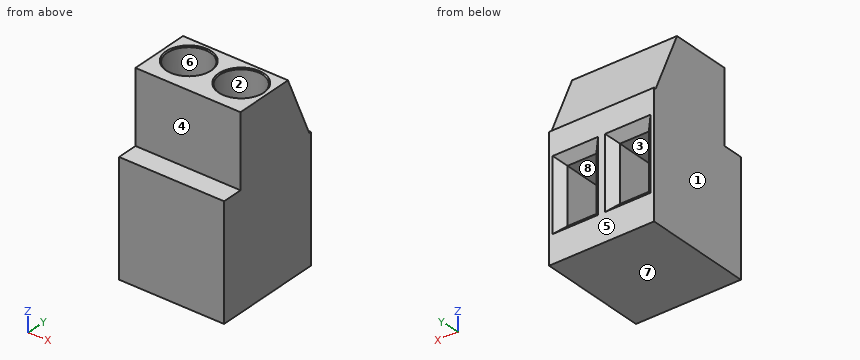
```python
from build123d import *

# Parameters (mm, degrees)
PAD_DEPTH       = 10.16
SKETCH001_R     = 2.1
POCKET_DEPTH    = 3
SKETCH002_W     = 5.4
SKETCH002_H     = 2.8
POCKET001_DEPTH = 8
CHAMFER_SIZE    = 0.8
CHAMFER001_SIZE = 0.1


with BuildPart() as part:
    # Sketch → Pad (new body)
    with BuildSketch(Plane.YZ):
        Polygon((-5.3, 0), (5.3, 0), (5.3, 12), (5.1, 12), (2.5, 18), (-3.3, 18), (-3.3, 11), (-5.3, 11), align=None)
    extrude(amount=PAD_DEPTH)

    # Sketch001 (on Face5 of Pad) → Pocket (cut)
    with BuildSketch(Plane(origin=(0, 0, 18), x_dir=(0, -1, 0), z_dir=(0, 0, 1))):
        with Locations((0, 2.54)):
            Circle(SKETCH001_R)
        with Locations((0, 7.62)):
            Circle(SKETCH001_R)
    extrude(amount=-POCKET_DEPTH, mode=Mode.SUBTRACT)

    # Sketch002 (on Face3 of Pocket) → Pocket001 (cut)
    with BuildSketch(Plane.ZX.offset(5.3)):
        with Locations((6.2, 7.62)):
            Rectangle(SKETCH002_W, SKETCH002_H)
        with Locations((6.2, 2.54)):
            Rectangle(SKETCH002_W, SKETCH002_H)
    extrude(amount=-POCKET001_DEPTH, mode=Mode.SUBTRACT)

    # Chamfer
    chamfer_edges = [part.edges().sort_by_distance(p)[0] for p in [
        (6.22, 5.3, 6.2),
        (7.62, 5.3, 8.9),
        (9.02, 5.3, 6.2),
        (7.62, 5.3, 3.5),
        (3.94, 5.3, 6.2),
        (2.54, 5.3, 8.9),
        (1.14, 5.3, 6.2),
        (2.54, 5.3, 3.5),
    ]]
    chamfer(chamfer_edges, length=CHAMFER_SIZE)

    # Chamfer001
    chamfer001_edges = [part.edges().sort_by_distance(p)[0] for p in [
        (7.62, 2.1, 18),
        (2.54, 2.1, 18),
    ]]
    chamfer(chamfer001_edges, length=CHAMFER001_SIZE)


solid = part.part
```
Geometry check sheet. Reference: the model listing, model coordinates, mm. Face numbers are marked on the shaded views. A direction names the side the tool comes from. Round coordinates to 2 decimals unless told otherwise and drop trailing zeros. Order: outer loops, then holes, each group sorted by start corner. A loop starts at its lowest first (then second) coordinate and runs counter-clockwise, first axis right, second up. Notation, with made-up numbers: (-27.5, 13) - (-10.5, 13) arc R24 cw to (-10.5, 29) - close; hole circle Ø7 at (-20, -13). An arc over 180 degrees is marked (long way). Use a Markdown table: item, result. Add a question column.
(1) Material ranges on line 1 along X through (y, z) = (-0.75, 7.5); line 2 along X through (y, z) = (0, 15.8); line 3 along Z through (x, y) = (1.25, -2.5), recorded low to high. Write a range as [from, to].
(2) Tool access check on the marked faces 1, 2, 3, 4 and 5. Record the directions out of +Z, -Z, +X, -X, +Y, -Y that give a thin tool (end or side, any length) a straight path to the whole face; none if there is none.
(3) Sectioned sample at A-A, the plane z = 4. Enter the section's corners in (x, y).
(4) Depth check by flat-ended pin: pin 1 (0.8 mm diameter, centred on x = 2, z = 6, fed in from +Y); pin 2 (0.8 mm diameter, centred on x = 2.5, y = 2, fed in from -Z); pin 3 (2 mm diameter, centred on x = 3, y = 0.5, fed in from +Z). Enter the tip coordinate at first touch or a pass-through.
(5) Sectioned sample at C-C, the plane x = 2.54. Enter the section's corners in (y, z).
(6) Sectioned sample at D-D, the plane y = -4.5. Enter the section's corners in (x, z).
(7) Sectioned sample at B-B, the plane y = 0. Enter the section's corners in (x, z).
(8) Release check for a two-part mould opening along Z. For the marked faces 6, 7 and 8 record: pulls with the +Z half, pulls with the -Z half, needs draft (parallel to the pull), parting line crosses it, or undercut.
Answers below:
| question | item | result |
|---|---|---|
| 1 | line 1 | [0, 1.14], [3.94, 6.22], [9.02, 10.16] |
| 1 | line 2 | [0, 0.44], [4.64, 5.52], [9.72, 10.16] |
| 1 | line 3 | [0, 3.5], [8.9, 18] |
| 2 | face 1 | +Z, -Z, -X, +Y, -Y |
| 2 | face 2 | +Z |
| 2 | face 3 | +Y |
| 2 | face 4 | +Z, +X, -X, -Y |
| 2 | face 5 | +Z, -Z, +X, -X, +Y |
| 3 | outline | (0, -5.3) - (10.16, -5.3) - (10.16, 5.3) - (9.82, 5.3) - (9.02, 4.5) - (9.02, -2.7) - (6.22, -2.7) - (6.22, 4.5) - (5.42, 5.3) - (4.74, 5.3) - (3.94, 4.5) - (3.94, -2.7) - (1.14, -2.7) - (1.14, 4.5) - (0.34, 5.3) - (0, 5.3) - close |
| 4 | pin 1 | y = -2.7 |
| 4 | pin 2 | z = 0 |
| 4 | pin 3 | z = 15 |
| 5 | outline | (-5.3, 0) - (5.3, 0) - (5.3, 2.7) - (4.5, 3.5) - (-2.7, 3.5) - (-2.7, 8.9) - (4.5, 8.9) - (5.3, 9.7) - (5.3, 12) - (5.1, 12) - (2.5, 18) - (2.2, 18) - (2.1, 17.9) - (2.1, 15) - (-2.1, 15) - (-2.1, 17.9) - (-2.2, 18) - (-3.3, 18) - (-3.3, 11) - (-5.3, 11) - close |
| 6 | outline | (0, 0) - (10.16, 0) - (10.16, 11) - (0, 11) - close |
| 7 | outline | (0, 0) - (10.16, 0) - (10.16, 18) - (9.82, 18) - (9.72, 17.9) - (9.72, 15) - (5.52, 15) - (5.52, 17.9) - (5.42, 18) - (4.74, 18) - (4.64, 17.9) - (4.64, 15) - (0.44, 15) - (0.44, 17.9) - (0.34, 18) - (0, 18) - close; hole (1.14, 3.5) - (3.94, 3.5) - (3.94, 8.9) - (1.14, 8.9) - close; hole (6.22, 3.5) - (9.02, 3.5) - (9.02, 8.9) - (6.22, 8.9) - close |
| 8 | face 6 | needs draft |
| 8 | face 7 | pulls with the -Z half |
| 8 | face 8 | undercut |
